```python
from build123d import *

# Parameters (mm, degrees)
SKETCH1_R                   = 11.1125
BOSS_EXTRUDE1_DEPTH         = 22.225
SKETCH2_R                   = 15.875
BOSS_EXTRUDE2_DEPTH         = 2.54
F_1_4_0_25_DIAMETER_HOLE1_D = 6.35


with BuildPart() as part:
    # Sketch1 → Boss-Extrude1 (new body)
    with BuildSketch(Plane(origin=(0, 0, 0), x_dir=(1, 0, 0), z_dir=(0, 1, 0))):
        Circle(SKETCH1_R)
    extrude(amount=BOSS_EXTRUDE1_DEPTH)

    # Sketch2 → Boss-Extrude2 (add)
    with BuildSketch(Plane(origin=(0, 22.225, 0), x_dir=(1, 0, 0), z_dir=(0, 1, 0))):
        Circle(SKETCH2_R)
    extrude(amount=-BOSS_EXTRUDE2_DEPTH)

    # 1/4 (0.25) Diameter Hole1 (through all)
    with Locations(Plane(origin=(0, 22.225, 0), x_dir=(1, 0, 0), z_dir=(0, 1, 0))):
        with Locations((0, 0)):
            Hole(F_1_4_0_25_DIAMETER_HOLE1_D / 2)


solid = part.part
```
Model file for the job. Use its own axes, mm. A direction names the side the tool comes from. Coordinates: 2 decimals unless noted, no trailing zeros. Loops run counter-clockwise (first coordinate to the right, second up) from the corner with the lowest first, then second, coordinate; pieces in that order, holes last. Notation, with made-up numbers: (30, 68) - (55, 68) arc R24 ccw to (55, 89) - close; hole circle Ø4 at (2, 15). An arc over 180 degrees is marked (long way). Answer as a JSON object with one key per item and string values. Group by question number.
(1) Cut at B-B (z = 0). Give the cut face in (x, y) (1 decimal).
(2) Tool access for faces 1 (the face through (-11, 19.685, 3)), 2 (the face through (0, 22.225, -4)): list every direction of +Z, -Z, +X, -X, +Y, -Y with a clear straight run to the whole face (end or side of a thin tool).
(3) Probe line 1 along Z through (x, y) = (0, 15) (1 decimal); line 2 along X through (y, z) = (10.25, -1.5); line 3 along X through (y, z) = (20.25, -0.5). List the from-to ranges inside material, lowest first.
(4) Cut at C-C (z = -6.5). Give the cut face in (x, y) (3 decimals), then the cut area to 3 significant figures.
(5) Cut at A-A (x = 0). Give the cut face in (y, z) (1 decimal).
(6) Flat gauge pins, fed straight in: pin 1 (10 mm diameter, centred on x = -4, y = 19.5, fed in from -Z) (3 decimals); pin 2 (1 mm diameter, centred on x = -6, y = 4.5, fed in from -Z); pin 3 (2 mm diameter, centred on y = 11.5, z = 6, fed in from -X); pin 4 (1 mm diameter, centred on x = -5, y = 14.5, fed in from +Z). Where does each tip first touch, or does it go through?
(7) Two-plate mould, pull along X, no slides. Class faces 3 (the face through (-3.441, 20.973, 15.497)), 4 (the face through (-3, 0, 2)), 5 (the face through (0.69, 10.96, 3.1)): released by +X, released by -X, zero draft, split by the parting line, or undercut.
Geometry says:
{
 "1": {"outline": "(-15.9, 19.7) - (-11.1, 19.7) - (-11.1, 0) - (-3.2, 0) - (-3.2, 22.2) - (-15.9, 22.2) - close; (3.2, 0) - (11.1, 0) - (11.1, 19.7) - (15.9, 19.7) - (15.9, 22.2) - (3.2, 22.2) - close"},
 "2": {"face 1": "-Y", "face 2": "+Z, -Z, +X, -X, +Y"},
 "3": {"line 1": "z = -11.1 to -3.2, 3.2 to 11.1", "line 2": "x = -11.01 to -2.8, 2.8 to 11.01", "line 3": "x = -15.87 to -3.14, 3.14 to 15.87"},
 "4": {"outline": "(-14.483, 19.685) - (-9.013, 19.685) - (-9.013, 0) - (9.013, 0) - (9.013, 19.685) - (14.483, 19.685) - (14.483, 22.225) - (-14.483, 22.225) - close", "area": "428 mm^2"},
 "5": {"outline": "(0, -11.1) - (19.7, -11.1) - (19.7, -15.9) - (22.2, -15.9) - (22.2, -3.2) - (0, -3.2) - close; (0, 3.2) - (22.2, 3.2) - (22.2, 15.9) - (19.7, 15.9) - (19.7, 11.1) - (0, 11.1) - close"},
 "6": {"pin 1": "stops at z = -15.875", "pin 2": "stops at z = -9.66", "pin 3": "stops at x = -9.92", "pin 4": "stops at z = 10.16"},
 "7": {"face 3": "split by the parting line", "face 4": "zero draft", "face 5": "undercut"}
}
